from build123d import *

# Parameters (mm, degrees)
F0_W     = 762
F0_H     = 660.4
F1_DEPTH = 76.2
F2_T     = -3.81
F3_R     = 31.75
F4_DEPTH = 3.811


with BuildPart() as f1:
    # F0 (on Top) → F1 (new body)
    with BuildSketch(Plane.XY):
        with Locations((-71.169143, 69.000456)):
            Rectangle(F0_W, F0_H)
    extrude(amount=F1_DEPTH)

    # F2
    f2_openings = [f1.faces().sort_by_distance(p)[0] for p in [
        (-71.169143, 69.000456, 76.2),
    ]]
    offset(amount=F2_T, openings=f2_openings)

    # F3 (on face) → F4 (cut, through all)
    with BuildSketch(Plane.XY.offset(3.81)):
        with Locations((153.620857, -65.028675)):
            Circle(F3_R)
    extrude(amount=-F4_DEPTH, mode=Mode.SUBTRACT)


solid = f1.part
Source: CAD feature listing. Evaluate the final solid. Frame: model axes, mm. A direction names the side the tool comes from. Give positions to 0.01 mm unless a question says otherwise; leave off trailing zeros. Write each loop counter-clockwise with the first axis right and the second up, starting at its lowest first coordinate (ties: lowest second). Pieces come first, ordered by that corner, then holes. Notation, with made-up numbers: M -17,81 L -6,81 A19 ccw -6,118 Z; hole C 72.25,18.25 d7. An arc over 180 degrees is marked long. Answer as a JSON object with one key per item and string values.
Q1. Contact query for a flat-ended pin moving along its axis: P1, Ø10, axis at x = -279, y = -184.5, coming from the +Z side. Output: stop coordinate, or through.
Geometry check:
{"P1": "stops at z = 3.81"}
Q2. Cut plane D-D, the plane x = 168. Return the cut outline in (y, z).
Geometry check:
{"outline": "M -261.2,0 L -93.34,0 L -93.34,3.81 L -257.39,3.81 L -257.39,76.2 L -261.2,76.2 Z; M -36.72,0 L 399.2,0 L 399.2,76.2 L 395.39,76.2 L 395.39,3.81 L -36.72,3.81 Z"}
Q3. Mould query, pull axis Y, two halves, no side actions, for faces 1 (the face through (182.95, -77.19, 1.93)), 2 (the face through (-77, 74, 0)), 3 (the face through (-77, -261.2, 38)). Classes: +Y half, -Y half, draft (parallel to the pull), parting line (faces both ways), or undercut.
Geometry check:
{"face 1": "undercut", "face 2": "draft", "face 3": "-Y half"}
Q4. Cut plane C-C, the plane y = 351.5. Return the cut outline in (x, z), then the cut area to 3 significant figures.
Geometry check:
{"outline": "M -452.17,0 L 309.83,0 L 309.83,76.2 L 306.02,76.2 L 306.02,3.81 L -448.36,3.81 L -448.36,76.2 L -452.17,76.2 Z", "area": "3,450 mm^2"}
Q5. Cut plane A-A, the plane z = 56.5. Return the cut outline in (x, y).
Geometry check:
{"outline": "M -452.17,-261.2 L 309.83,-261.2 L 309.83,399.2 L -452.17,399.2 Z; hole M -448.36,-257.39 L 306.02,-257.39 L 306.02,395.39 L -448.36,395.39 Z"}
Q6. Cut plane B-B, the plane x = -376. Return the cut outline in (y, z), then the cut area to 3 significant figures.
Geometry check:
{"outline": "M -261.2,0 L 399.2,0 L 399.2,76.2 L 395.39,76.2 L 395.39,3.81 L -257.39,3.81 L -257.39,76.2 L -261.2,76.2 Z", "area": "3,070 mm^2"}
Q7. Access query for faces 4 (the face through (309.831, 64, 38)), 5 (the face through (-76, -257.39, 39)). Directions: +Z, -Z, +X, -X, +Y, -Y. A direction counts if a zero-diameter tool reaches every point of the face in a straight line with its end or side. Return the directions, or none.
Geometry check:
{"face 4": "+Z, -Z, +X, +Y, -Y", "face 5": "+Z"}
Q8. Ray query, line 1 along Y through (x, z) = (193, 69.5); line 2 along X through (y, z) = (294, 53); line 3 along Z through (x, y) = (35, 178.5). Return the intervals inside material, ascending.
Geometry check:
{"line 1": "y = -261.2 to -257.39, 395.39 to 399.2", "line 2": "x = -452.17 to -448.36, 306.02 to 309.83", "line 3": "z = 0 to 3.81"}
